Source: CAD feature listing. Evaluate the final solid. Frame: model axes, mm. Face numbers are marked on the shaded views. A direction names the side the tool comes from. Give positions to 0.01 mm unless a question says otherwise; leave off trailing zeros. Order: outer loops, then holes, each group sorted by start corner. A loop starts at its lowest first (then second) coordinate and runs counter-clockwise, first axis right, second up. Notation, with made-up numbers: (74, 23.25) -> (112, 23.25) arc R26 cw to (112, 56.25) -> close; hole circle Ø5 at (-38, -37). An arc over 180 degrees is marked (long way). Use one line per item in the form item = value. Start each with the question number.
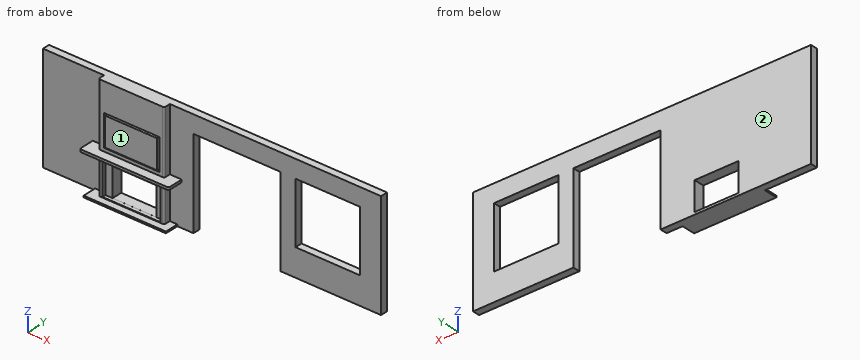
from build123d import *

# Parameters (mm, degrees)
F0_W           = 36.2768345653
F0_H           = 34.5578843861
F1_DEPTH       = 4
F3_DEPTH       = 60
F4_W           = 24.767242372
F4_H           = 16.1051880568
F5_DEPTH       = 25
F6_DEPTH       = 28.2239038497
F7_W           = 32.4881970882
F7_H           = 19.8430884629
F7_W_2         = 24.767242372
F7_H_2         = 16.1051880568
F8_DEPTH       = 1.9791987725
F9_W           = 36.9808363765
F9_H           = 4
F10_DEPTH      = 0.9402669966
F11_W          = 29.2263142765
F11_H          = 16.1546287127
F12_DEPTH      = 0.5
F13_W          = 31.2264300883
F13_H          = 17.6170864142
F13_W_2        = 29.2263142765
F13_H_2        = 16.1546287127
F14_DEPTH      = 1.5
F15_W          = 7.6713270694
F15_H          = 1.4258362353
F15_W_2        = 34.9808363765
F15_W_3        = 7.3478365541
F16_DEPTH      = 5
F16_DEPTH_BACK = 4.8303701915
F17_R          = 1


with BuildPart() as f1:
    # F0 (on Front) → F1 (new body)
    with BuildSketch(Plane.XZ):
        Polygon((95.8462816477, 30.5567865909), (-94.1537183523, 30.5567865909), (-94.1537183523, -29.4432134091), (-9.5833106827, -29.4432134091), (-9.5833106827, 20.6685056415), (39.3904383138, 20.6685056415), (39.3904383138, -29.4432134091), (95.8462816477, -29.4432134091), align=None)
        with Locations((65.9178723932, 3.2533946408)):
            Rectangle(F0_W, F0_H, mode=Mode.SUBTRACT)
    extrude(amount=F1_DEPTH)

    # F2 (on face) → F3 (join)
    with BuildSketch(Plane(origin=(0, 0, -29.4432134091), x_dir=(1, 0, 0), z_dir=(0, 0, -1))):
        with BuildLine():
            Line((-59.8266199231, 6.7806394547), (-59.8266199231, 4))
            Line((-59.8266199231, 4), (-22.8457835466, 4))
            Line((-22.8457835466, 4), (-22.8457835466, 6.7806394547))
            ThreePointArc((-22.8457835466, 6.7806394547), (-23.1386767654, 7.4877462359), (-23.8457835466, 7.7806394547))
            Line((-23.8457835466, 7.7806394547), (-58.8266199231, 7.7806394547))
            ThreePointArc((-58.8266199231, 7.7806394547), (-59.5337267043, 7.4877462359), (-59.8266199231, 6.7806394547))
        make_face()
    extrude(amount=-F3_DEPTH)

    # F4 (on face) → F5 (join)
    with BuildSketch(Plane.XZ):
        with Locations((-41.1277525127, -20.0668377802)):
            Rectangle(F4_W, F4_H)
    extrude(amount=F5_DEPTH)

    # F6 (cut): a face of the model
    f6_faces = [f1.faces().sort_by_distance(p)[0] for p in [
        (-41.1277525127, -25, -20.0668377802),
    ]]
    extrude(f6_faces, amount=-F6_DEPTH, mode=Mode.SUBTRACT)

    # F7 (on face) → F8 (cut)
    with BuildSketch(Plane.XZ.offset(7.7806394547)):
        with Locations((-41.1744564772, -18.2105200365)):
            Rectangle(F7_W, F7_H)
        with Locations((-41.1277525127, -20.0668377802)):
            Rectangle(F7_W_2, F7_H_2, mode=Mode.SUBTRACT)
    extrude(amount=-F8_DEPTH, mode=Mode.SUBTRACT)

    # F9 (on face) → F10 (join)
    with BuildSketch(Plane(origin=(0, 0, -29.4432134091), x_dir=(1, 0, 0), z_dir=(0, 0, -1))):
        Polygon((-64.8606717587, 11.7061249912), (-64.8606717587, 0), (-59.8266199231, 0), (-59.8266199231, 4), (-22.8457835466, 4), (-22.8457835466, 0), (-18.5923743993, 0), (-18.5923743993, 11.7061249912), align=None)
        with Locations((-41.3362017348, 2)):
            Rectangle(F9_W, F9_H)
    extrude(amount=-F10_DEPTH)

    # F11 (on face) → F12 (join)
    with BuildSketch(Plane.XZ.offset(7.7806394547)):
        with Locations((-41.1195810884, 5.75606036)):
            Rectangle(F11_W, F11_H)
    extrude(amount=F12_DEPTH)

    # F13 (on face) → F14 (cut)
    with BuildSketch(Plane.XZ.offset(7.7806394547)):
        with Locations((-41.1195810884, 5.75606036)):
            Rectangle(F13_W, F13_H)
        with Locations((-41.1195810884, 5.75606036)):
            Rectangle(F13_W_2, F13_H_2, mode=Mode.SUBTRACT)
    extrude(amount=-F14_DEPTH, mode=Mode.SUBTRACT)

    # F15 (on face) → F16 (join, two sides)
    with BuildSketch(Plane.XZ.offset(7.7806394547)) as f16_sk:
        with Locations((-20.0101200119, -5.6498679332)):
            Rectangle(F15_W, F15_H)
        with Locations((-41.3362017348, -5.6498679332)):
            Rectangle(F15_W_2, F15_H)
        with Locations((-62.5005382001, -5.6498679332)):
            Rectangle(F15_W_3, F15_H)
    extrude(amount=F16_DEPTH)
    extrude(f16_sk.sketch, amount=-F16_DEPTH_BACK)

    # F17
    f17_edges = [f1.edges().sort_by_distance(p)[0] for p in [
        (-16.174456, -12.780639, -5.649868),
        (-66.174456, -12.780639, -5.649868),
    ]]
    fillet(f17_edges, radius=F17_R)


solid = f1.part
1) Cut plane D-D, the plane z = -21.5. Return the cut outline in (x, y), plus the area to 4 significant figures.
2) Cut plane C-C, the plane y = -10. Return the cut outline in (x, z).
3) Cut plane A-A, the plane z = 5. Return the cut outline in (x, y), plus the area to 3 significant figures.
4) Reachability of the marked faces 1 and 2 from +Z, -Z, +X, -X, +Y, -Y: full face, straight path, thin tool, end or side. Return the list, or none.
5) Pin query (flat end, axial travel): pin 1 (10 mm diameter, centred on x = -37, z = -19.5, fed in from -Y); pin 2 (5 mm diameter, centred on y = -7, z = -8, fed in from -X); pin 3 (0.6 mm diameter, centred on y = -7.5, z = 3, fed in from -X); pin 4 (1.4 mm diameter, centred on y = -6, z = -21.5, fed in from -X). Return the tip coordinate at first contact, or that it passes through.
6) Material intervals for probe 1 along X at (y, z) = (-1.5, -6.5); probe 2 along X at (y, z) = (-7.5, 6.5); probe 3 along Z at (x, y) = (-49.5, -2.5), sorted ascending.
Output values:
q1.outline = (-94.15, -4) -> (-59.83, -4) -> (-59.83, -6.78) arc R1 ccw to (-58.83, -7.78) -> (-57.42, -7.78) -> (-57.42, -5.8) -> (-53.51, -5.8) -> (-53.51, 0) -> (-94.15, 0) -> close; (-28.74, -5.8) -> (-24.93, -5.8) -> (-24.93, -7.78) -> (-23.85, -7.78) arc R1 ccw to (-22.85, -6.78) -> (-22.85, -4) -> (-9.58, -4) -> (-9.58, 0) -> (-28.74, 0) -> close; (39.39, -4) -> (95.85, -4) -> (95.85, 0) -> (39.39, 0) -> close
q1.area = 495.5 mm^2
q2.outline = (-66.17, -6.36) -> (-16.17, -6.36) -> (-16.17, -4.94) -> (-66.17, -4.94) -> close; (-64.86, -29.44) -> (-18.59, -29.44) -> (-18.59, -28.5) -> (-64.86, -28.5) -> close
q3.outline = (-94.15, -4) -> (-59.83, -4) -> (-59.83, -6.78) arc R1 ccw to (-58.83, -7.78) -> (-56.73, -7.78) -> (-56.73, -6.28) -> (-55.73, -6.28) -> (-55.73, -8.28) -> (-26.51, -8.28) -> (-26.51, -6.28) -> (-25.51, -6.28) -> (-25.51, -7.78) -> (-23.85, -7.78) arc R1 ccw to (-22.85, -6.78) -> (-22.85, -4) -> (-9.58, -4) -> (-9.58, 0) -> (-94.15, 0) -> close; (39.39, -4) -> (47.78, -4) -> (47.78, 0) -> (39.39, 0) -> close; (84.06, -4) -> (95.85, -4) -> (95.85, 0) -> (84.06, 0) -> close
q3.area = 570 mm^2
q4.face_1 = +Z, +X, -X, -Y
q4.face_2 = +Z, -Z, +X, -X, +Y
q5.pin_1 = through
q5.pin_2 = -66.17
q5.pin_3 = -59.73
q5.pin_4 = -59.83
q6.probe_1 = -94.15 to -9.58, 39.39 to 47.78, 84.06 to 95.85
q6.probe_2 = -59.52 to -56.73, -55.73 to -26.51, -25.51 to -23.15
q6.probe_3 = -29.44 to -28.12, -12.01 to 30.56
